Here's how the part is built. I have some questions about the finished solid (model axes, mm). Face numbers are marked on the shaded views. A direction names the side the tool comes from. Give positions to 0.01 mm unless a question says otherwise; leave off trailing zeros. Loops run counter-clockwise (first coordinate to the right, second up) from the corner with the lowest first, then second, coordinate; pieces in that order, holes last. Notation, with made-up numbers: (38, -22.75) - (84, -22.75) arc R22 cw to (84, 5.25) - close; hole circle Ø8 at (-2.5, 5.25). An arc over 180 degrees is marked (long way). Use a Markdown table: item, result.
from build123d import *

# Parameters (mm, degrees)
TAIL_START              = -21.9
TAIL_BLOCK_DEPTH        = 50.15
NOSE_START              = 22.2
SKETCH2_R               = 8
NOSE_WALL_X_DEPTH       = 4
NOSE_START_2            = -21.9
NOSE_WALLS_DEPTH        = 44.3
HEAD_START              = 8.2
SKETCH4_W               = 21
SKETCH4_H               = 8
HEAD_SERVO_LEDGES_DEPTH = 14.2
TAB_START               = 8
SKETCH5_R               = 1.7
TAB_BOLT_HOLES_DEPTH    = 9.2
TAB_START_2             = 11.7
TAB_NUT_SLOTS_DEPTH     = 2.7
MOUNT_START             = -22.1
SKETCH7_R               = 1.7
MOUNT_BOLT_HOLES_DEPTH  = 50.55
COVER_START             = -22.1
SKETCH8_R               = 1.7
COVER_BOLT_HOLE_DEPTH   = 14.1
D_SIDE_START            = 18.9
D_SIDE_NUT_SLOTS_DEPTH  = 2.7
I_SIDE_START            = -17.5
I_SIDE_NUT_SLOTS_DEPTH  = 2.7
COVER_START_2           = -16.4
COVER_NUT_SLOT_DEPTH    = 2.7
LEAD_START              = -22.1
SKETCH12_W              = 8
SKETCH12_H              = 14.6
LEAD_CHANNEL_DEPTH      = 14.1


with BuildPart() as part:
    # Sketch1 → Tail block (new body)
    with BuildSketch(Plane(origin=(0, 0, 0), x_dir=(0, 0, -1), z_dir=(1, 0, 0)).offset(TAIL_START)):
        with BuildLine():
            Line((-1.5, 271.5), (-1.5, 279.5))
            ThreePointArc((-1.5, 279.5), (-2.378679656, 281.621320344), (-4.5, 282.5))
            Line((-4.5, 282.5), (-23.5, 282.5))
            ThreePointArc((-23.5, 282.5), (-25.621320344, 281.621320344), (-26.5, 279.5))
            Line((-26.5, 279.5), (-26.5, 271.5))
            ThreePointArc((-26.5, 271.5), (-25.621320344, 269.378679656), (-23.5, 268.5))
            Line((-23.5, 268.5), (-4.5, 268.5))
            ThreePointArc((-4.5, 268.5), (-2.378679656, 269.378679656), (-1.5, 271.5))
        make_face()
    extrude(amount=TAIL_BLOCK_DEPTH)

    # Sketch2 → Nose wall +X (add)
    with BuildSketch(Plane(origin=(0, 0, 0), x_dir=(0, 0, -1), z_dir=(1, 0, 0)).offset(NOSE_START)):
        with BuildLine():
            Line((-0.7, 282.3), (-0.7, 336))
            ThreePointArc((-0.7, 336), (-2.457359313, 340.242640687), (-6.7, 342))
            Line((-6.7, 342), (-21.3, 342))
            ThreePointArc((-21.3, 342), (-25.542640687, 340.242640687), (-27.3, 336))
            Line((-27.3, 336), (-27.3, 282.3))
            Line((-27.3, 282.3), (-0.7, 282.3))
        make_face()
        with Locations((-14, 320.5)):
            Circle(SKETCH2_R, mode=Mode.SUBTRACT)
    extrude(amount=NOSE_WALL_X_DEPTH)

    # Sketch3 → Nose walls (add)
    with BuildSketch(Plane(origin=(0, 0, 0), x_dir=(0, 0, -1), z_dir=(1, 0, 0)).offset(NOSE_START_2)):
        with BuildLine():
            Line((-0.7, 282.3), (-0.7, 336))
            ThreePointArc((-0.7, 336), (-2.457359313, 340.242640687), (-6.7, 342))
            Line((-6.7, 342), (-21.3, 342))
            ThreePointArc((-21.3, 342), (-25.542640687, 340.242640687), (-27.3, 336))
            Line((-27.3, 336), (-27.3, 282.3))
            Line((-27.3, 282.3), (-24.3, 282.3))
            Line((-24.3, 282.3), (-24.3, 337))
            ThreePointArc((-24.3, 337), (-24.007106781, 337.707106781), (-23.3, 338))
            Line((-23.3, 338), (-4.7, 338))
            ThreePointArc((-4.7, 338), (-3.992893219, 337.707106781), (-3.7, 337))
            Line((-3.7, 337), (-3.7, 282.3))
            Line((-3.7, 282.3), (-0.7, 282.3))
        make_face()
    extrude(amount=NOSE_WALLS_DEPTH)

    # Sketch4 → Head servo ledges (add)
    with BuildSketch(Plane(origin=(0, 0, 0), x_dir=(0, 0, -1), z_dir=(1, 0, 0)).offset(HEAD_START)):
        with Locations((-14, 334.9)):
            Rectangle(SKETCH4_W, SKETCH4_H)
        with Locations((-14, 285.4)):
            Rectangle(SKETCH4_W, SKETCH4_H)
    extrude(amount=HEAD_SERVO_LEDGES_DEPTH)

    # Sketch5 → Tab bolt holes (cut)
    with BuildSketch(Plane(origin=(0, 0, 0), x_dir=(0, 0, -1), z_dir=(1, 0, 0)).offset(TAB_START)):
        with Locations((-9, 334.9)):
            Circle(SKETCH5_R)
        with Locations((-19, 334.9)):
            Circle(SKETCH5_R)
        with Locations((-9, 285.4)):
            Circle(SKETCH5_R)
        with Locations((-19, 285.4)):
            Circle(SKETCH5_R)
    extrude(amount=TAB_BOLT_HOLES_DEPTH, mode=Mode.SUBTRACT)

    # Sketch6 → Tab nut slots (cut)
    with BuildSketch(Plane(origin=(0, 0, 0), x_dir=(0, 0, -1), z_dir=(1, 0, 0)).offset(TAB_START_2)):
        Polygon((-6.05, 333.196816706), (-6.05, 336.603183294), (-9, 338.306366588), (-11.95, 336.603183294), (-11.95, 333.196816706), (-11.95, 330.4), (-6.05, 330.4), align=None)
        Polygon((-16.05, 333.196816706), (-16.05, 336.603183294), (-19, 338.306366588), (-21.95, 336.603183294), (-21.95, 333.196816706), (-21.95, 330.4), (-16.05, 330.4), align=None)
        Polygon((-11.95, 287.103183294), (-11.95, 283.696816706), (-9, 281.993633412), (-6.05, 283.696816706), (-6.05, 287.103183294), (-6.05, 289.9), (-11.95, 289.9), align=None)
        Polygon((-21.95, 287.103183294), (-21.95, 283.696816706), (-19, 281.993633412), (-16.05, 283.696816706), (-16.05, 287.103183294), (-16.05, 289.9), (-21.95, 289.9), align=None)
    extrude(amount=TAB_NUT_SLOTS_DEPTH, mode=Mode.SUBTRACT)

    # Sketch7 → Mount bolt holes (cut)
    with BuildSketch(Plane(origin=(0, 0, 0), x_dir=(0, 0, -1), z_dir=(1, 0, 0)).offset(MOUNT_START)):
        with Locations(Location((-7, 274.5, 0), (0, 0, 180))):
            Circle(SKETCH7_R)
        with Locations(Location((-21, 274.5, 0), (0, 0, 180))):
            Circle(SKETCH7_R)
    extrude(amount=MOUNT_BOLT_HOLES_DEPTH, mode=Mode.SUBTRACT)

    # Sketch8 → Cover bolt hole (cut)
    with BuildSketch(Plane(origin=(0, 0, 0), x_dir=(0, 0, -1), z_dir=(1, 0, 0)).offset(COVER_START)):
        with Locations((-14, 340)):
            Circle(SKETCH8_R)
    extrude(amount=COVER_BOLT_HOLE_DEPTH, mode=Mode.SUBTRACT)

    # Sketch9 → D-side nut slots (cut)
    with BuildSketch(Plane(origin=(0, 0, 0), x_dir=(0, 0, -1), z_dir=(1, 0, 0)).offset(D_SIDE_START)):
        Polygon((-5.296816706, 277.45), (-8.703183294, 277.45), (-10.406366588, 274.5), (-8.703183294, 271.55), (-5.296816706, 271.55), (-1, 271.55), (-1, 277.45), align=None)
        Polygon((-22.703183294, 271.55), (-19.296816706, 271.55), (-17.593633412, 274.5), (-19.296816706, 277.45), (-22.703183294, 277.45), (-27, 277.45), (-27, 271.55), align=None)
    extrude(amount=D_SIDE_NUT_SLOTS_DEPTH, mode=Mode.SUBTRACT)

    # Sketch10 → I-side nut slots (cut)
    with BuildSketch(Plane(origin=(0, 0, 0), x_dir=(0, 0, -1), z_dir=(1, 0, 0)).offset(I_SIDE_START)):
        Polygon((-5.296816706, 277.45), (-8.703183294, 277.45), (-10.406366588, 274.5), (-8.703183294, 271.55), (-5.296816706, 271.55), (-1, 271.55), (-1, 277.45), align=None)
        Polygon((-22.703183294, 271.55), (-19.296816706, 271.55), (-17.593633412, 274.5), (-19.296816706, 277.45), (-22.703183294, 277.45), (-27, 277.45), (-27, 271.55), align=None)
    extrude(amount=I_SIDE_NUT_SLOTS_DEPTH, mode=Mode.SUBTRACT)

    # Sketch11 → Cover nut slot (cut)
    with BuildSketch(Plane(origin=(0, 0, 0), x_dir=(0, 0, -1), z_dir=(1, 0, 0)).offset(COVER_START_2)):
        Polygon((-16.95, 341.703183294), (-16.95, 338.296816706), (-14, 336.593633412), (-11.05, 338.296816706), (-11.05, 341.703183294), (-11.05, 342.5), (-16.95, 342.5), align=None)
    extrude(amount=COVER_NUT_SLOT_DEPTH, mode=Mode.SUBTRACT)

    # Sketch12 → Lead channel (cut)
    with BuildSketch(Plane(origin=(0, 0, 0), x_dir=(0, 0, -1), z_dir=(1, 0, 0)).offset(LEAD_START)):
        with Locations((-14, 275.5)):
            Rectangle(SKETCH12_W, SKETCH12_H)
    extrude(amount=LEAD_CHANNEL_DEPTH, mode=Mode.SUBTRACT)


solid = part.part
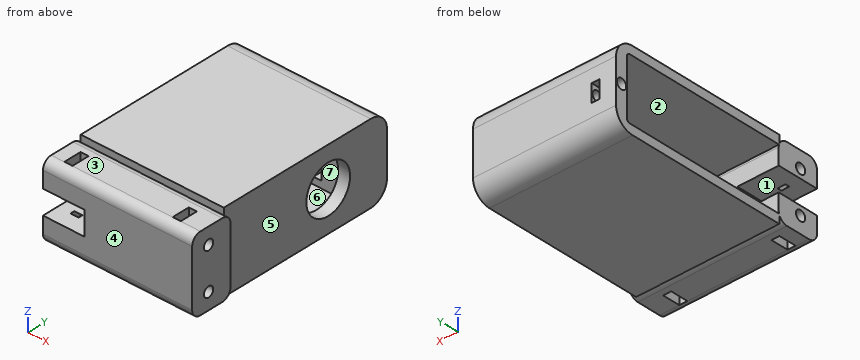
(1) Suppose I cut it at B-B on x = 9. Write out the boundary of the cut face in (y, z), plus the area to 3 significant figures.
A:
| item | result |
|---|---|
| outline | (268.5, 4.5) arc R3 ccw to (271.5, 1.5) - (279.5, 1.5) arc R3 ccw to (282.3, 3.42) - (282.3, 0.7) - (336, 0.7) arc R6 ccw to (342, 6.7) - (342, 21.3) arc R6 ccw to (336, 27.3) - (282.3, 27.3) - (282.3, 24.58) arc R3 ccw to (279.5, 26.5) - (271.5, 26.5) arc R3 ccw to (268.5, 23.5) - close; hole circle Ø3.4 at (274.5, 7); hole circle Ø3.4 at (274.5, 21); hole circle Ø3.4 at (285.4, 9); hole circle Ø3.4 at (285.4, 19); hole (289.4, 3.7) - (330.9, 3.7) - (330.9, 24.3) - (289.4, 24.3) - close; hole circle Ø3.4 at (334.9, 9); hole circle Ø3.4 at (334.9, 19) |
| area | 1,000 mm2 |
(2) On a 3-axis mill with a long thin cutter (end or side, diameter ignored), from which of +Z, -Z, +X, -X, +Y, -Y can I reach the whole of each face in a straight line? I mean the marked faces 1, 2 and 3. Say none if no direction works.
A:
| item | result |
|---|---|
| face 1 | -X, -Y |
| face 2 | -X |
| face 3 | +Z, +X, -X, -Y |
(3) Will these pins go through, and if not, where does the flat tip stop? pin 1 (7 mm diameter, centred on x = -17.5, y = 272.5, fed in from -Z); pin 2 (5 mm diameter, centred on y = 327, z = 11, fed in from -X); pin 3 (1.5 mm diameter, centred on y = 282.5, z = 12, fed in from -X).
A:
| item | result |
|---|---|
| pin 1 | z = 1.5 |
| pin 2 | x = 22.2 |
| pin 3 | x = -8 |
(4) Suppose I cut it at D-D on x = 2. Write out the boundary of the cut face in (y, z).
A:
| item | result |
|---|---|
| outline | (268.5, 4.5) arc R3 ccw to (271.5, 1.5) - (279.5, 1.5) arc R3 ccw to (282.3, 3.42) - (282.3, 0.7) - (336, 0.7) arc R6 ccw to (342, 6.7) - (342, 21.3) arc R6 ccw to (336, 27.3) - (282.3, 27.3) - (282.3, 24.58) arc R3 ccw to (279.5, 26.5) - (271.5, 26.5) arc R3 ccw to (268.5, 23.5) - close; hole circle Ø3.4 at (274.5, 7); hole circle Ø3.4 at (274.5, 21); hole (282.39, 3.7) - (337, 3.7) arc R1 ccw to (338, 4.7) - (338, 23.3) arc R1 ccw to (337, 24.3) - (282.39, 24.3) arc R3 cw to (282.5, 23.5) - (282.5, 4.5) arc R3 cw to start |
(5) If I drill on line 1 (Z direction, x = 15.85, y = 334.9); line 2 (Y direction, x = 16.25, z = 9); line 3 (Z direction, x = 6.5, y = 297), over which ranges is the centre line in solid material (lowest first)?
A:
| item | result |
|---|---|
| line 1 | 0.7 to 7.3, 10.7 to 17.3, 20.7 to 27.3 |
| line 2 | 268.5 to 283.7, 287.1 to 289.4, 330.9 to 333.2, 336.6 to 342 |
| line 3 | 0.7 to 3.7, 24.3 to 27.3 |
(6) Suppose I cut it at A-A on x = 25. Write out the boundary of the cut face in (y, z).
A:
| item | result |
|---|---|
| outline | (268.5, 4.5) arc R3 ccw to (271.5, 1.5) - (279.5, 1.5) arc R3 ccw to (282.3, 3.42) - (282.3, 0.7) - (336, 0.7) arc R6 ccw to (342, 6.7) - (342, 21.3) arc R6 ccw to (336, 27.3) - (282.3, 27.3) - (282.3, 24.58) arc R3 ccw to (279.5, 26.5) - (271.5, 26.5) arc R3 ccw to (268.5, 23.5) - close; hole circle Ø3.4 at (274.5, 7); hole circle Ø3.4 at (274.5, 21); hole circle Ø16 at (320.5, 14) |
(7) We'd pull the mould along Y, two halves only. Please class the marked faces 4, 5, 6 and 7: pulls with the +Y half, pulls with the -Y half, needs draft (parallel to the pull), parting line crosses it, or undercut.
A:
| item | result |
|---|---|
| face 4 | pulls with the -Y half |
| face 5 | needs draft |
| face 6 | undercut |
| face 7 | undercut |
(8) Suppose I cut it at C-C on y = 322.5. Write out the boundary of the cut face in (x, z).
A:
| item | result |
|---|---|
| outline | (-21.9, 0.7) - (26.2, 0.7) - (26.2, 6.25) - (22.2, 6.25) - (22.2, 3.7) - (-21.9, 3.7) - close; (-21.9, 24.3) - (22.2, 24.3) - (22.2, 21.75) - (26.2, 21.75) - (26.2, 27.3) - (-21.9, 27.3) - close |
